The model under review builds one solid part; all positions refer to its coordinate system, in mm. Face numbers are marked on the shaded views. A direction names the side the tool comes from. Round coordinates to 2 decimals unless told otherwise and drop trailing zeros. Write each loop counter-clockwise with the first axis right and the second up, starting at its lowest first coordinate (ties: lowest second). Pieces come first, ordered by that corner, then holes. Notation, with made-up numbers: (-14, 81) -> (39, 81) arc R22 cw to (39, 95) -> close; hole circle Ø9 at (86.5, 78.25). An arc over 180 degrees is marked (long way). Use CSV: the item, a comma, the result in double quotes. Start each with the question number.
1) Take a section at C-C, the plane y = -2. Give the boundary of the cut face in (x, z).
2) Machinability: for the marked faces 4, 5 and 6, which of the approach directions +Z, -Z, +X, -X, +Y, -Y give a long, thin tool a straight path to every point of the face, cutting with its end or side? Answer none if there is none.
3) Take a section at B-B, the plane x = 0. Give the boundary of the cut face in (y, z), then the cut area to 3 significant figures.
4) Take a section at A-A, the plane z = 0. Give the boundary of the cut face in (x, y).
5) Take a section at D-D, the plane y = 1.25. Give the boundary of the cut face in (x, z).
6) For pin 1 Ø1 at (x, y) = (0.5, 2.5) entering from -Z; pin 2 Ø1.1 at (y, z) = (3.5, 1.5) entering from +X; pin 3 Ø4 at (x, y) = (-2.5, 3.5) entering from +Z, all flat-tipped, find the tip position at first contact; note any pin that passes through.
7) Mouldability with a two-part tool opening along X and no side actions: class the marked faces 1, 2 and 3 as released by +X, released by -X, zero draft, split by the parting line, or undercut.
8) Wall thickness on probe 1 along Y at (x, z) = (2.75, 0.25); probe 2 along Y at (x, z) = (-2.5, -2.75); probe 3 along Y at (x, z) = (1, 0): over which ranges is each line inside the solid? List them lowest first. Write a range as [from, to].
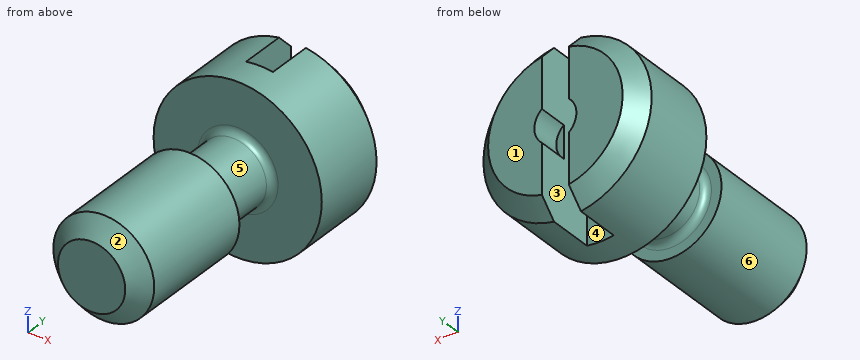
Autodesk Inventor part; units mm, degrees
ref_plane "YZ Plane" through (0, 0, 0) normal (1, 0, 0) x (0, 1, 0)
ref_plane "XZ Plane" through (0, 0, 0) normal (0, 1, 0) x (-1, 0, 0)
ref_plane "XY Plane" through (0, 0, 0) normal (0, 0, 1) x (1, 0, 0)
sketch "Sketch1" plane through (0, 0, 0) normal (0, 0, 1) x (1, 0, 0)
  line L0 (5, 0) -> (5, 5.5)
  line L1 (5, 5.5) -> (0, 5.5)
  line L2 (5, 0) -> (2, 0)
  line L3 (2, 0) -> (2, -4)
  line L4 (2, -4) -> (3, -4)
  line L5 (3, -4) -> (3, -12)
  line L6 (3, -12) -> (0, -12)
  line L7 (0, 5.5) -> (0, -12)
  point P0 (0, 0)
  dimension "d0" = 10
  dimension "d2" = 4
  dimension "d3" = 6
  dimension "d4" = 5.5
  dimension "d5" = 8
  dimension "d6" = 12
revolve "Вращение1" add sketch "Sketch1" angle 360 about axis through (0, 5.5, 0) along (0, -1, 0)
sketch "Sketch2" plane through (0, 5.5, 0) normal (0, 1, 0) x (1, 0, 0)
  circle A0 centre (0, 0) radius 5 construction
  circle A1 centre (0, 0) radius 1.25
  dimension "d31" = 2.5
extrude "Выдавливание1" cut sketch "Sketch2" against normal blind 1.8
chamfer "Фаска1" distance 1 angle 45 1 edges at (-5, 5.5, 0)
sketch "Sketch3" plane through (0, 0, 0) normal (0, 0, 1) x (1, 0, 0)
  line L0 (0, 0) -> (0, 5.5)
  line L1 (-2.3552, 0) -> (2.3552, 0) construction
  line L2 (-5, 5.5) -> (5, 5.5) construction
  line L3 (-0.8, 5.5) -> (0.8, 5.5)
  line L4 (0.8, 5.5) -> (0.8, 1.8)
  line L5 (0.8, 1.8) -> (-0.8, 1.8)
  line L6 (-0.8, 1.8) -> (-0.8, 5.5)
  dimension "d8" = 1.8
  dimension "d9" = 1.6
extrude "Выдавливание2" cut sketch "Sketch3" along normal through all both and the other way through all
fillet "Сопряжение1" radius 0.4 2 edges at (-2, 0, 0) (-2, -4, 0)
thread "Резьба1"
chamfer "Фаска2" distance 1 angle 45 1 edges at (-3, -12, 0)
equation "\"d31\" = d3_"
equation "\"d32\" = h3"
equation "\"d21\" = C1"
equation "\"d8\" = h2"
equation "\"d9\" = n"
equation "\"d12\" = R"
equation "\"d13\" = b"
equation "\"d15\" = C1"
equation "\"d0\" = D"
equation "\"d2\" = d1"
equation "\"d3\" = d_"
equation "\"d4\" = k1"
equation "\"d5\" = b"
equation "\"d6\" = l_"
equation "\"D\" = 10"
equation "\"d_\" = 6"
equation "\"l_\" = 12"
equation "\"b\" = 8"
equation "\"d1\" = 4"
equation "\"R\" = 0.4"
equation "\"C1\" = 1"
equation "\"h2\" = 1.8"
equation "\"n\" = 1.6"
equation "\"h3\" = 1.8"
equation "\"k1\" = 5.5"
equation "\"d3_\" = 2.5"
equation "\"G\" = l_ - b"
properties part number "Винт 3 M6-6gx12 ГОСТ 10336-80" material "Сталь, мягкая"
Values found:
1,outline,"circle Ø4 at (0, 0)"
2,face 4,"+Z, -Z, +Y"
2,face 5,"none"
2,face 6,"-Y"
3,outline,"(-12, -2) -> (-11, -3) -> (-4, -3) -> (-4, -2.4) arc R0.4 cw to (-3.6, -2) -> (-0.4, -2) arc R0.4 cw to (0, -2.4) -> (0, -5) -> (1.8, -5) -> (1.8, 5) -> (0, 5) -> (0, 2.4) arc R0.4 cw to (-0.4, 2) -> (-3.6, 2) arc R0.4 cw to (-4, 2.4) -> (-4, 3) -> (-11, 3) -> (-12, 2) -> close"
3,area,"81.1 mm²"
4,outline,"(-5, 0) -> (-2.4, 0) arc R0.4 cw to (-2, -0.4) -> (-2, -3.6) arc R0.4 cw to (-2.4, -4) -> (-3, -4) -> (-3, -11) -> (-2, -12) -> (2, -12) -> (3, -11) -> (3, -4) -> (2.4, -4) arc R0.4 cw to (2, -3.6) -> (2, -0.4) arc R0.4 cw to (2.4, 0) -> (5, 0) -> (5, 4.5) -> (4, 5.5) -> (1.25, 5.5) -> (1.25, 3.7) -> (0.8, 3.7) -> (0.8, 1.8) -> (-0.8, 1.8) -> (-0.8, 3.7) -> (-1.25, 3.7) -> (-1.25, 5.5) -> (-4, 5.5) -> (-5, 4.5) -> close"
5,outline,"circle Ø10 at (0, 0)"
6,pin 1,"z = -4.94"
6,pin 2,"x = 4.91"
6,pin 3,"z = 4.94"
7,face 1,"zero draft"
7,face 2,"split by the parting line"
7,face 3,"undercut"
8,probe 1,"[-11.24, -4], [0, 5.5]"
8,probe 2,"[0, 5.5]"
8,probe 3,"[-12, 3.7]"
